Source: three-view drawing plus pictorial views. Frame: mm from the lowest corner of the part. A direction names the side the tool comes from. Give positions to 0.01 mm unless a question says otherwise; leave off trailing zeros. Loops run counter-clockwise (first coordinate to the right, second up) from the corner with the lowest first, then second, coordinate; pieces in that order, holes last. Notation, with made-up numbers: (31, 36.5) -> (36, 36.5) arc R12 ccw to (36, 40.5) -> close; hole circle Ø4 at (75.25, 10). An arc over 180 degrees is marked (long way). Put each result on its own line as item: value.
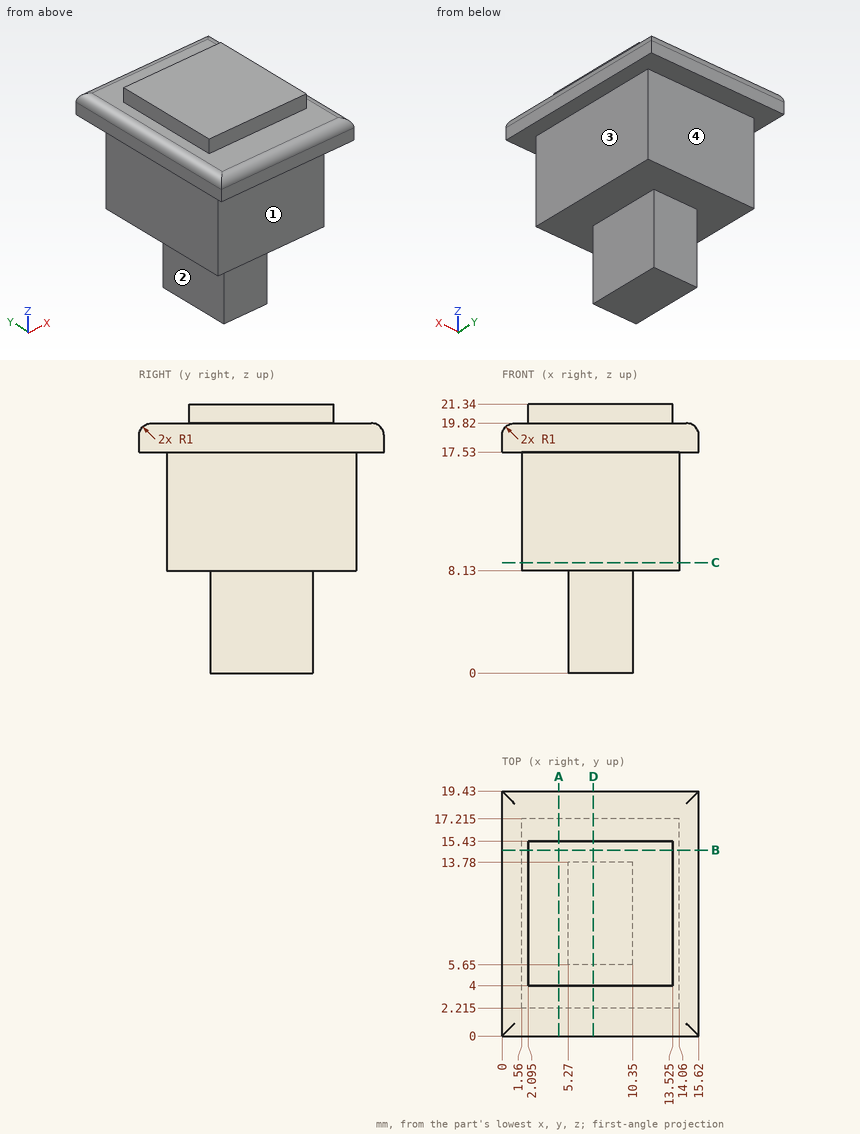
(1) Section A-A on x = 4.5. Return loops of the section in (y, z) (3 decimals), then the cut area to 3 significant figures.
Calculated:
outline: (0, 17.53) -> (2.215, 17.53) -> (2.215, 8.13) -> (17.215, 8.13) -> (17.215, 17.53) -> (19.43, 17.53) -> (19.43, 18.82) arc R1 ccw to (18.43, 19.82) -> (15.43, 19.82) -> (15.43, 21.34) -> (4, 21.34) -> (4, 19.82) -> (1, 19.82) arc R1 ccw to (0, 18.82) -> close
area: 202 mm²
(2) First-contact query: P1, Ø4.5, axis at x = 5, z = 11, coming from the -Y side (3 decimals); P2, Ø10, axis at y = 6.5, z = 9, coming from the -X side; P3, Ø1, axis at x = 12.5, z = 11, coming from the +Y side (3 decimals); P4, Ø2, axis at y = 15, z = 6.5, coming from the +X side. Flat tips, straight axial feed; report the tip coordinate or a pass-through.
Calculated:
P1: stops at y = 2.215
P2: stops at x = 1.56
P3: stops at y = 17.215
P4: passes through
(3) Line query: probe 1 along Z at (x, y) = (11.25, 13.5); probe 2 along Y at (x, z) = (11, 15.75) (3 decimals); probe 3 along X at (y, z) = (5.5, 11.75). Output: solid intervals per line, ascending. Write a range as from..to.
Calculated:
probe 1: z = 8.13..21.34
probe 2: y = 2.215..17.215
probe 3: x = 1.56..14.06
(4) Section C-C on z = 8.75. Return loops of the section in (x, y) (3 decimals), then the cut area to 4 significant figures.
Calculated:
outline: (1.56, 2.215) -> (14.06, 2.215) -> (14.06, 17.215) -> (1.56, 17.215) -> close
area: 187.5 mm²
(5) Section B-B on y = 14.75. Return loops of the section in (x, z) (3 decimals).
Calculated:
outline: (0, 17.53) -> (1.56, 17.53) -> (1.56, 8.13) -> (14.06, 8.13) -> (14.06, 17.53) -> (15.62, 17.53) -> (15.62, 18.82) arc R1 ccw to (14.62, 19.82) -> (13.525, 19.82) -> (13.525, 21.34) -> (2.095, 21.34) -> (2.095, 19.82) -> (1, 19.82) arc R1 ccw to (0, 18.82) -> close
(6) Section D-D on x = 7.25. Return loops of the section in (y, z) (3 decimals).
Calculated:
outline: (0, 17.53) -> (2.215, 17.53) -> (2.215, 8.13) -> (5.65, 8.13) -> (5.65, 0) -> (13.78, 0) -> (13.78, 8.13) -> (17.215, 8.13) -> (17.215, 17.53) -> (19.43, 17.53) -> (19.43, 18.82) arc R1 ccw to (18.43, 19.82) -> (15.43, 19.82) -> (15.43, 21.34) -> (4, 21.34) -> (4, 19.82) -> (1, 19.82) arc R1 ccw to (0, 18.82) -> close
(7) Reachability of the marked faces 1, 2, 3 and 4 from +Z, -Z, +X, -X, +Y, -Y: full face, straight path, thin tool, end or side. Return the list, or none.
Calculated:
face 1: -Z, +X, -X, -Y
face 2: -Z, -X, +Y, -Y
face 3: -Z, +X, +Y, -Y
face 4: -Z, +X, -X, +Y
